Could you check a few things on this drawing? It's one solid part, dimensions in mm from its lowest x, y, z. A direction names the side the tool comes from. Coordinates: 2 decimals unless noted, no trailing zeros. Order: outer loops, then holes, each group sorted by start corner. A loop starts at its lowest first (then second) coordinate and runs counter-clockwise, first axis right, second up. Notation, with made-up numbers: (3, 32) -> (23, 32) arc R8 cw to (23, 44) -> close; hole circle Ø5 at (-25, 79). An arc over 180 degrees is marked (long way). Answer as CSV lines item,"result".
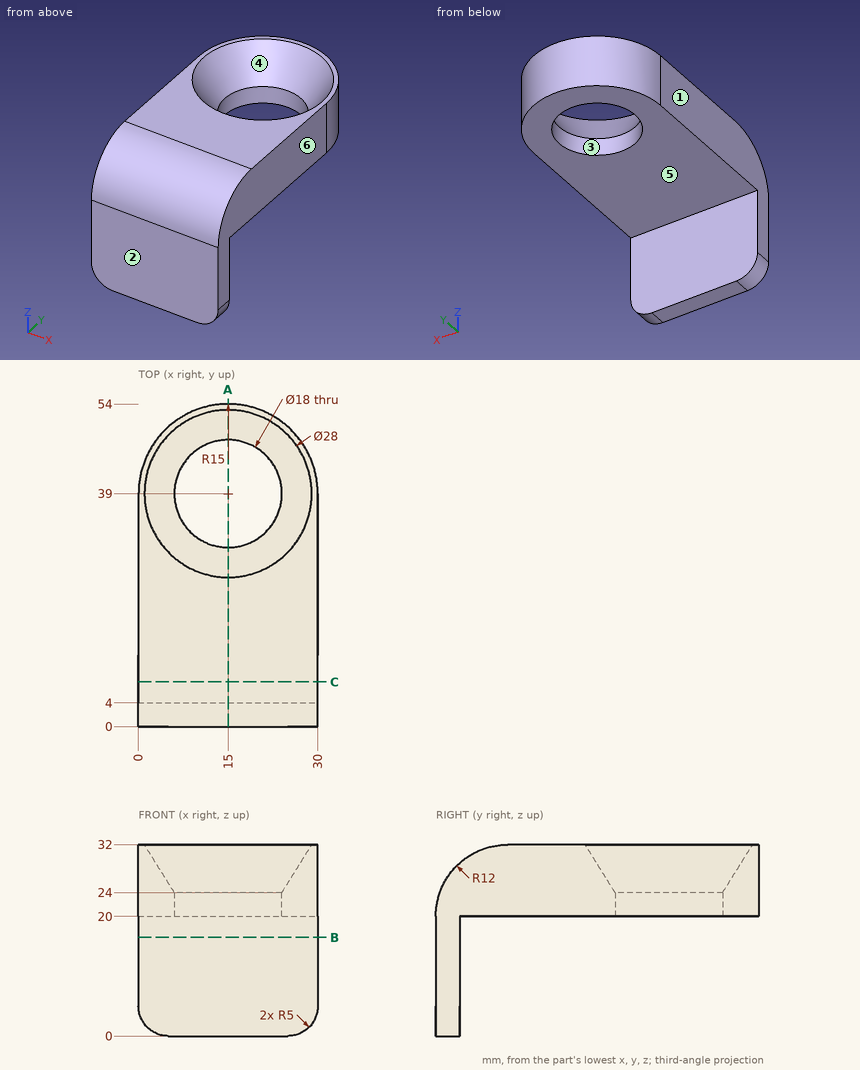
Q1. Imagine slicing it at A-A (x = 15). List the corners of the cut face in (y, z) for me, and give its area (3 significant figures).
Solution:
outline,"(0, 0) -> (4, 0) -> (4, 20) -> (30, 20) -> (30, 24) -> (25, 32) -> (12, 32) arc R12 ccw to (0, 20) -> close; (48, 20) -> (54, 20) -> (54, 32) -> (53, 32) -> (48, 24) -> close"
area,"441 mm2"
Q2. Imagine slicing it at B-B (z = 16.5). List the corners of the cut face in (x, y) for me.
Solution:
outline,"(0, 0) -> (30, 0) -> (30, 4) -> (0, 4) -> close"
Q3. For P1, Ø6, axis at x = 9, y = 7, coming from the +Z side; P2, Ø12, axis at x = 12, z = 9, coming from the +Y side; P3, Ø1.5, axis at x = 22, y = 30, coming from the -Z side, each with a flat end and sliding along its axis, tell me the tip position at first contact or that it passes through.
Solution:
P1,"z = 31.83"
P2,"y = 4"
P3,"z = 20"
Q4. We'd pull the mould along X, two halves only. Please class the marked faces 1, 2, 3 and 4: pulls with the +X half, pulls with the -X half, needs draft (parallel to the pull), parting line crosses it, or undercut.
Solution:
face 1,"pulls with the -X half"
face 2,"needs draft"
face 3,"undercut"
face 4,"undercut"
Q5. If I drill on line 1 (Y direction, x = 25.25, z = 17.5); line 2 (Z direction, x = 21, y = 26); line 3 (Y direction, x = 15, z = 22.05), over which ranges is the centre line in solid material (lowest first)?
Solution:
line 1,"0 to 4"
line 2,"20 to 32"
line 3,"0.18 to 30, 48 to 54"
Q6. Which directions (+Z, -Z, +X, -X, +Y, -Y) give clear straight access to the entire face, cutting with the end or side of a thin tool? Please do the marked faces 5 and 6.
Solution:
face 5,"-Z, +X, -X, +Y"
face 6,"+Z, -Z, +X, +Y, -Y"
Q7. Imagine slicing it at C-C (y = 7.5). List the corners of the cut face in (x, z) for me.
Solution:
outline,"(0, 20) -> (30, 20) -> (30, 31.12) -> (0, 31.12) -> close"
